Geometry: final body of the model. Coordinates: model frame, mm. A direction names the side the tool comes from. Give positions to 0.01 mm unless a question says otherwise; leave off trailing zeros. Write each loop counter-clockwise with the first axis right and the second up, starting at its lowest first coordinate (ties: lowest second). Pieces come first, ordered by that corner, then holes. Notation, with made-up numbers: (-12.5, 50.25) -> (23.5, 50.25) arc R14 cw to (23.5, 66.25) -> close; hole circle Ø10 at (13.5, -40). An arc over 180 degrees is marked (long way). Answer in a Markdown table with one row per item. Add a question column.
from build123d import *

# Parameters (mm, degrees)
F1_DEPTH  = 16
F2_W      = 70
F2_H      = 2
F3_DEPTH  = 2
F4_W      = 50
F4_H      = 10
F4_H_2    = 2
F5_DEPTH  = 2
F6_R      = 1
F9_DEPTH  = 2
F11_DEPTH = 40.001
F12_R     = 2
F13_DEPTH = 40.001
F12_R_2   = 3
F14_DEPTH = 8
F15_R     = 2
F16_DEPTH = 6


with BuildPart() as f1:
    # F0 (on Front) → F1 (new body)
    with BuildSketch(Plane.XZ):
        with BuildLine():
            ThreePointArc((-78.2553477167, -4.5), (-82.7553477167, 0), (-78.2553477167, 4.5))
            Line((-78.2553477167, 4.5), (15.7446522833, 4.5))
            Line((15.7446522833, 4.5), (15.7446522833, 6.5))
            Line((15.7446522833, 6.5), (-78.2553477167, 6.5))
            ThreePointArc((-78.2553477167, 6.5), (-84.7553477167, 0), (-78.2553477167, -6.5))
            Line((-78.2553477167, -6.5), (-63.5440570211, -6.5))
            ThreePointArc((-63.5440570211, -6.5), (-61.6242210154, -7.1947386892), (-60.5935745764, -8.9571801926))
            ThreePointArc((-60.5935745764, -8.9571801926), (-45.7228537684, -41.2574258057), (-17.207438999, -62.5016091164))
            ThreePointArc((-17.207438999, -62.5016091164), (-13.2164359403, -63.5063644425), (-10.3436688231, -66.4533710204))
            Line((-10.3436688231, -66.4533710204), (-8.58552102, -65.5))
            ThreePointArc((-8.58552102, -65.5), (-12.0235125852, -61.888485404), (-16.8125554919, -60.5))
            ThreePointArc((-16.8125554919, -60.5), (-44.2937887319, -39.8437899922), (-58.6265862799, -8.5953003211))
            ThreePointArc((-58.6265862799, -8.5953003211), (-60.3443303449, -5.6578978153), (-63.5440570211, -4.5))
            Line((-63.5440570211, -4.5), (-78.2553477167, -4.5))
        make_face()
    extrude(amount=F1_DEPTH)

    # F2 (on face) → F3 (join)
    with BuildSketch(Plane.XY.offset(6.5)):
        with Locations((-19.2553477167, -17)):
            Rectangle(F2_W, F2_H)
    extrude(amount=-F3_DEPTH)

    # F4 (on face) → F5 (join)
    with BuildSketch(Plane.XZ.offset(18)):
        with Locations((-9.2553477167, -0.5)):
            Rectangle(F4_W, F4_H)
        with Locations((-9.2553477167, 5.5)):
            Rectangle(F4_W, F4_H_2)
    extrude(amount=F5_DEPTH)

    # F6
    f6_edges = [f1.edges().sort_by_distance(p)[0] for p in [
        (-9.255348, -20, 6.5),
        (-9.255348, -18, 4.5),
    ]]
    fillet(f6_edges, radius=F6_R)

    # F7: F1 across face


with BuildPart() as f1_1:
    add(f1.part)
    add(f1.part.mirror(Plane(origin=(-41.9712348224, 0, -13.8038322502), x_dir=(1, 0, 0), z_dir=(0, 1, 0))))

    # F8 (on face) → F9 (cut)
    with BuildSketch(Plane.XY.offset(6.5)):
        with BuildLine():
            Line((15.7446522833, 12), (-44.2553477167, 12))
            ThreePointArc((-44.2553477167, 12), (-56.2553477167, 0), (-44.2553477167, -12))
            Line((-44.2553477167, -12), (15.7446522833, -12))
            Line((15.7446522833, -12), (15.7446522833, 12))
        make_face()
    extrude(amount=-F9_DEPTH, mode=Mode.SUBTRACT)

    # F10 (on face) → F11 (cut, through all)
    with BuildSketch(Plane.XZ.offset(20)):
        with BuildLine():
            ThreePointArc((-28.2553477167, 3), (-31.2553477167, 0), (-28.2553477167, -3))
            Line((-28.2553477167, -3), (-8.2553477167, -3))
            ThreePointArc((-8.2553477167, -3), (-5.2553477167, 0), (-8.2553477167, 3))
            Line((-8.2553477167, 3), (-28.2553477167, 3))
        make_face()
    extrude(amount=-F11_DEPTH, mode=Mode.SUBTRACT)

    # F12 (on face) → F13 (cut, through all)
    with BuildSketch(Plane.XZ.offset(20)):
        with Locations((1.7446522833, 0.5)):
            Circle(F12_R)
    extrude(amount=-F13_DEPTH, mode=Mode.SUBTRACT)

    # F12 (on face) → F14 (join)
    with BuildSketch(Plane.XZ.offset(20)):
        with Locations((1.7446522833, 0.5)):
            Circle(F12_R_2)
        with Locations((1.7446522833, 0.5)):
            Circle(F12_R, mode=Mode.SUBTRACT)
    extrude(amount=-F14_DEPTH)

    # F15 (on face) → F16 (join)
    with BuildSketch(Plane.XZ.offset(-18)):
        with BuildLine():
            ThreePointArc((1.7446522833, 3.5), (-0.3766680603, -1.6213203436), (4.7446522833, 0.5))
            ThreePointArc((4.7446522833, 0.5), (3.8659726268, 2.6213203436), (1.7446522833, 3.5))
        make_face()
        with Locations((1.7446522833, 0.5)):
            Circle(F15_R, mode=Mode.SUBTRACT)
    extrude(amount=F16_DEPTH)


solid = f1_1.part
Q1. Line query: probe 1 along Y at (x, z) = (1, 2.5); probe 2 along X at (y, z) = (-14, 0); probe 3 along Z at (x, y) = (-10.5, 17). Output: solid intervals per line, ascending. Write a range as from..to.
Q2. Section A-A on x = -71.5. Return loops of the section in (y, z).
Q3. Section C-C on x = -22. Return loops of the section in (y, z).
Q4. Access query for faces 4 (the flat face through (-44, -18, 6)), 5 (the flat face through (-71, 0, -6.5)), 6 (the cylindrical face through (-56.252, 0.264, 5.514)), 7 (the flat face through (-18, 19, -3)). Directions: +Z, -Z, +X, -X, +Y, -Y. A direction counts if a zero-diameter tool reaches every point of the face in a straight line with its end or side. Return the directions, or none.
Q5. Section B-B on y = 0. Return loops of the section in (x, z).
Q6. Pull-direction query (Y, two-part tool) for faces 1 (the flat face through (-55, 16, -22)), 2 (the flat face through (4, 12, 0)), 3 (the cylindrical face through (-11.963, -0.224, -61.925)); classes: +Y half, -Y half, draft (parallel to the pull), parting line (faces both ways), or undercut.
Q7. Contact query for flat-ended pins moving along their axis: pin 1 Ø4.5 at (x, y) = (-71, -4) entering from -Z; pin 2 Ø1.6 at (y, z) = (16.5, 6) entering from -X; pin 3 Ø1 at (y, z) = (-14.5, -19) entering from +X. Output: stop coordinate, or through.
Q8. Section D-D on z = -59. Return loops of the section in (x, y).
Checks:
| question | item | result |
|---|---|---|
| 1 | probe 1 | -20..-12, 12..20 |
| 1 | probe 2 | -84.76..-82.76, -1.21..-0.19, 3.68..4.7 |
| 1 | probe 3 | 4.5..6.5 |
| 2 | outline | (-16, -6.5) -> (16, -6.5) -> (16, -4.5) -> (-16, -4.5) -> close; (-16, 4.5) -> (16, 4.5) -> (16, 6.5) -> (-16, 6.5) -> close |
| 3 | outline | (-20, -5.5) -> (-18, -5.5) -> (-18, -3) -> (-20, -3) -> close; (-20, 3) -> (-18, 3) -> (-18, 3.5) arc R1 cw to (-17, 4.5) -> (-12, 4.5) -> (-12, 6.5) -> (-19, 6.5) arc R1 ccw to (-20, 5.5) -> close; (-16, -60.32) -> (16, -60.32) -> (16, -58.07) -> (-16, -58.07) -> close; (12, 4.5) -> (17, 4.5) arc R1 cw to (18, 3.5) -> (18, 3) -> (20, 3) -> (20, 5.5) arc R1 ccw to (19, 6.5) -> (12, 6.5) -> close; (18, -5.5) -> (20, -5.5) -> (20, -3) -> (18, -3) -> close |
| 4 | face 4 | +Z, -Z, -X, -Y |
| 4 | face 5 | -Z, -X, +Y, -Y |
| 4 | face 6 | +Z, +X |
| 4 | face 7 | +Y, -Y |
| 5 | outline | (-78.26, -6.5) -> (-63.54, -6.5) arc R3 cw to (-60.59, -8.96) arc R72 ccw to (-17.21, -62.5) arc R7.56 cw to (-10.34, -66.45) -> (-8.59, -65.5) arc R9.56 ccw to (-16.81, -60.5) arc R70 cw to (-58.63, -8.6) arc R5 ccw to (-63.54, -4.5) -> (-78.26, -4.5) arc R4.5 cw to (-78.26, 4.5) -> (-56.26, 4.5) -> (-56.26, 6.5) -> (-78.26, 6.5) arc R6.5 ccw to start |
| 6 | face 1 | +Y half |
| 6 | face 2 | undercut |
| 6 | face 3 | draft |
| 7 | pin 1 | z = -6.5 |
| 7 | pin 2 | x = -81.91 |
| 7 | pin 3 | x = -55.69 |
| 8 | outline | (-24.51, -16) -> (-20.15, -16) -> (-20.15, 16) -> (-24.51, 16) -> close |
